```python
from build123d import *

# Parameters (mm, degrees)
F1_DEPTH = 7
F2_R     = 1.5


with BuildPart() as f1:
    # F0 (on Top) → F1 (new body)
    with BuildSketch(Plane.XY):
        with BuildLine():
            ThreePointArc((8.367497, -7.140378), (0, -11), (-8.367497, -7.140378))
            Line((-8.367497, -7.140378), (-13.881214, -10.323724))
            ThreePointArc((-13.881214, -10.323724), (-13.40799, -12.134855), (-13.248711, -14))
            ThreePointArc((-13.248711, -14), (-20.443614, -24.320912), (-32.616208, -21.140378))
            Line((-32.616208, -21.140378), (-42.30127, -26.732051))
            Line((-42.30127, -26.732051), (42.30127, -26.732051))
            Line((42.30127, -26.732051), (32.616208, -21.140378))
            ThreePointArc((32.616208, -21.140378), (18.748711, -23.526279), (13.881214, -10.323724))
            Line((13.881214, -10.323724), (8.367497, -7.140378))
        make_face()
    extrude(amount=F1_DEPTH)

    # F2
    f2_edges = [f1.edges().sort_by_distance(p)[0] for p in [
        (-42.30127, -26.732051, 3.5),
        (42.30127, -26.732051, 3.5),
    ]]
    fillet(f2_edges, radius=F2_R)


solid = f1.part
```
CAD build for the part. Positions are in the model's coordinates, mm. Coordinates: 2 decimals unless noted, no trailing zeros. Order: outer loops, then holes, each group sorted by start corner. A loop starts at its lowest first (then second) coordinate and runs counter-clockwise, first axis right, second up. Notation, with made-up numbers: (23, -2) - (38, -2) arc R26 ccw to (38, 14) - close; hole circle Ø2 at (81.5, 50). An arc over 180 degrees is marked (long way). Use a Markdown table: item, result. Add a question column.
(1) Saw through at D-D (y = -13). Give the cut face in (x, z), then the cut area to 3 significant figures.
(2) Saw through at B-B (y = -22.25). Give the cut face in (x, z), then the cut area to 3 significant figures.
(3) Flat gauge pins, fed straight in: pin 1 (3 mm diameter, centred on x = 16, z = 6, fed in from +Y); pin 2 (8 mm diameter, centred on x = 25.5, y = -19, fed in from -Z); pin 3 (4 mm diameter, centred on y = -13.5, z = 1.5, fed in from -X). Where does each tip first touch, or does it go through?
(4) Saw through at C-C (x = -25). Give the cut face in (y, z).
(5) Saw through at A-A (z = 2.5). Give the cut face in (x, y).
(6) Pull direction X, two halves, no side cores. Call faces 1 (the face through (35.069, -22.556, 3.451)), 2 (the face through (0, -11, 3)), 3 (the face through (-1, -19, 0)): +X half, -X half, draft (parallel to the pull), parting line (faces both ways), or undercut.
(7) Drill centre lines: line 1 along X through (y, z) = (-13.75, 3.5); line 2 along X through (y, z) = (-23.75, 4.25); line 3 along Y through (x, z) = (-29, 4). Where is each one in solid material? Low to high. Write a range as [from, to].
Solved:
| question | item | result |
|---|---|---|
| 1 | outline | (-13.29, 0) - (13.29, 0) - (13.29, 7) - (-13.29, 7) - close |
| 1 | area | 186 mm² |
| 2 | outline | (-34.54, 0) - (-31.52, 0) - (-31.52, 7) - (-34.54, 7) - close; (-16.97, 0) - (16.97, 0) - (16.97, 7) - (-16.97, 7) - close; (31.52, 0) - (34.54, 0) - (34.54, 7) - (31.52, 7) - close |
| 2 | area | 280 mm² |
| 3 | pin 1 | stops at y = -19.1 |
| 3 | pin 2 | passes through |
| 3 | pin 3 | stops at x = -13.54 |
| 4 | outline | (-26.73, 0) - (-24.97, 0) - (-24.97, 7) - (-26.73, 7) - close |
| 5 | outline | (-37.45, -23.93) arc R1.5 ccw to (-36.7, -26.73) - (36.7, -26.73) arc R1.5 ccw to (37.45, -23.93) - (32.62, -21.14) arc R11 cw to (13.88, -10.32) - (8.37, -7.14) arc R11 cw to (-8.37, -7.14) - (-13.88, -10.32) arc R11 cw to (-13.25, -14) arc R11 cw to (-32.62, -21.14) - close |
| 6 | face 1 | +X half |
| 6 | face 2 | undercut |
| 6 | face 3 | draft |
| 7 | line 1 | x = [-13.25, 13.25] |
| 7 | line 2 | x = [-37.14, -29.34], [-19.16, 19.16], [29.34, 37.14] |
| 7 | line 3 | y = [-26.73, -23.92] |
